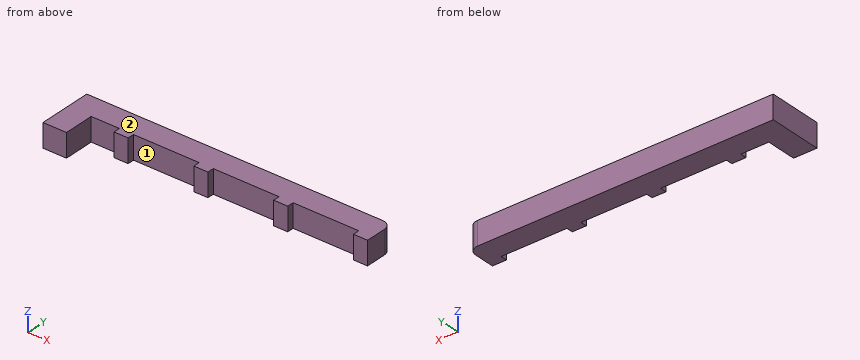
Autodesk Inventor part; units mm, degrees
ref_plane "YZ Plane" through (0, 0, 0) normal (1, 0, 0) x (0, 1, 0)
ref_plane "XZ Plane" through (0, 0, 0) normal (0, 1, 0) x (-1, 0, 0)
ref_plane "XY Plane" through (0, 0, 0) normal (0, 0, 1) x (1, 0, 0)
sketch "Эскиз1" plane through (0, 0, 0) normal (0, 1, 0) x (-1, 0, 0)
  line L0 (0, 0) -> (3, 0)
  line L1 (3, 0) -> (3, -5)
  line L2 (3, -5) -> (0, -5)
  line L3 (0, -5) -> (0, 0)
  line L4 (17, 0) -> (20, 0)
  line L5 (20, 0) -> (20, -5)
  line L6 (20, -5) -> (17, -5)
  line L7 (17, -5) -> (17, 0)
  line L8 (34, 0) -> (37, 0)
  line L9 (37, 0) -> (37, -5)
  line L10 (37, -5) -> (34, -5)
  line L11 (34, -5) -> (34, 0)
  line L12 (51, 0) -> (54, 0)
  line L13 (54, 0) -> (54, -5)
  line L14 (54, -5) -> (51, -5)
  line L15 (51, -5) -> (51, 0)
  dimension "d0" = 3
  dimension "d1" = 5
  dimension "d3" = 3
  dimension "d4" = 5
  dimension "d6" = 3
  dimension "d7" = 5
  dimension "d9" = 3
  dimension "d10" = 5
extrude "Выдавливание1" add sketch "Эскиз1" along normal blind 1.4
sketch "Эскиз2" plane through (0, 1.4, 0) normal (0, 1, 0) x (1, 0, 0)
  line L0 (0, 0) -> (-65, 0)
  line L1 (-65, 0) -> (-65, 5)
  line L2 (-65, 5) -> (0, 5)
  line L3 (0, 5) -> (0, 0)
  line L4 (-65, 0) -> (-60, 0)
  line L5 (-60, 5) -> (-65, 5)
  line L6 (-65, 5) -> (-65, 0)
  dimension "d14" = 65
extrude "Выдавливание2" add sketch "Эскиз2" along normal blind 5
fillet "Сопряжение1" radius 2 1 edges at (0, 6.4, -2.5)
sketch "Эскиз4" plane through (0, 1.4, 0) normal (0, -1, 0) x (1, 0, 0)
  line L0 (-65, 0) -> (-2, 0)
  line L1 (-65, 0) -> (-60, 0)
  line L2 (-60, 0) -> (-60, -5)
  line L3 (-60, -5) -> (-65, -5)
  line L4 (-65, -5) -> (-65, 0)
  point P0 (0, 0)
  dimension "d23" = 5
  dimension "d24" = 5
extrude "Выдавливание3" add sketch "Эскиз4" along normal blind 6.5
properties part number "Bus_copper_top" material "Медь"
The listing builds one solid part. Answer for the finished solid, in the listing's coordinates (mm). Face numbers are marked on the shaded views. A direction names the side the tool comes from. Give positions to 0.01 mm unless a question says otherwise; leave off trailing zeros. Loops run counter-clockwise (first coordinate to the right, second up) from the corner with the lowest first, then second, coordinate; pieces in that order, holes last. Notation, with made-up numbers: M 66,-33.5 L 79,-33.5 A29 cw 79,-9.5 Z; hole C 48.5,-9.5 d9. An arc over 180 degrees is marked long. One line per item, written item: value.
1. Find the intervals of material crossed by probe 1 along X at (y, z) = (1, -2.95); probe 2 along X at (y, z) = (-1.5, -3.4); probe 3 along Y at (x, z) = (-39.5, -2.05), in increasing order.
Found:
probe 1: -65 to -60, -54 to -51, -37 to -34, -20 to -17, -3 to 0
probe 2: -65 to -60
probe 3: 1.4 to 6.4
2. For the marked faces 1 and 2, determine the directions among +Z, -Z, +X, -X, +Y, -Y from which every point of the face is accessible in a straight line to the end or side of a thin tool.
Found:
face 1: +Z, -Z, -Y
face 2: +Z, +X, -X, +Y, -Y
3. Section A-A on z = -1.6 is taken. Determine the outline of the cut face in (x, y).
Found:
outline: M -65,-5.1 L -60,-5.1 L -60,1.4 L -54,1.4 L -54,0 L -51,0 L -51,1.4 L -37,1.4 L -37,0 L -34,0 L -34,1.4 L -20,1.4 L -20,0 L -17,0 L -17,1.4 L -3,1.4 L -3,0 L 0,0 L 0,4.4 A2 ccw -2,6.4 L -65,6.4 Z
4. Each of these flat-tipped pins is pushed along its axis until it touches: P1, Ø2.5, axis at x = -1.5, z = -2, coming from the -Y side; P2, Ø1.5, axis at x = -13, z = -1.5, coming from the -Y side. Where does it stop, or does it pass through?
Found:
P1: y = 0
P2: y = 1.4
5. Section B-B on x = -55.5 is taken. Determine the outline of the cut face in (y, z), plus the area to 3 significant figures.
Found:
outline: M 1.4,-5 L 6.4,-5 L 6.4,0 L 1.4,0 Z
area: 25.0 mm^2
6. Section C-C on y = -4 is taken. Determine the outline of the cut face in (x, z).
Found:
outline: M -65,-5 L -60,-5 L -60,0 L -65,0 Z
